from build123d import *

# Parameters (mm, degrees)
SKETCH2_W               = 9.652
SKETCH2_H               = 3.048
SKETCH2_W_2             = 3.048
SKETCH2_H_2             = 35.052
BOSS_EXTRUDE1_DEPTH     = 77.882279
SKETCH3_W               = 25.4
SKETCH3_H               = 76.2
SKETCH3_W_2             = 19.304
SKETCH3_H_2             = 70.104
BOSS_EXTRUDE2_DEPTH     = 50
CUT_EXTRUDE1_DEPTH      = 1
CUT_EXTRUDE1_DEPTH_BACK = 77.2
SKETCH5_W               = 25.4
SKETCH5_H               = 76.2
SKETCH5_W_2             = 19.304
SKETCH5_H_2             = 70.104
BOSS_EXTRUDE3_DEPTH     = 50
CUT_EXTRUDE2_DEPTH      = 1
CUT_EXTRUDE2_DEPTH_BACK = 77.2


with BuildPart() as part:
    # Sketch2 → Boss-Extrude1 (new body)
    with BuildSketch(Plane.XY):
        Polygon((-12.7, 0), (-9.652, 0), (-9.652, 35.052), (-9.652, 38.1), (-12.7, 38.1), align=None)
        with Locations((-4.826, 36.576)):
            Rectangle(SKETCH2_W, SKETCH2_H)
        Polygon((0, 38.1), (0, 35.052), (9.652, 35.052), (9.652, 0), (12.7, 0), (12.7, 38.1), align=None)
        with Locations((11.176, -17.526)):
            Rectangle(SKETCH2_W_2, SKETCH2_H_2)
        Polygon((-9.652, -35.052), (-9.652, 0), (-12.7, 0), (-12.7, -38.1), (0, -38.1), (0, -35.052), align=None)
        Polygon((9.652, -35.052), (0, -35.052), (0, -38.1), (12.7, -38.1), (12.7, -35.052), align=None)
    extrude(amount=BOSS_EXTRUDE1_DEPTH)

    # Sketch3 → Boss-Extrude2 (add)
    with BuildSketch(Plane(origin=(0, 0, 0), x_dir=(-1, 0, 0), z_dir=(0, 0, -1))):
        Rectangle(SKETCH3_W, SKETCH3_H)
        Rectangle(SKETCH3_W_2, SKETCH3_H_2, mode=Mode.SUBTRACT)
    extrude(amount=BOSS_EXTRUDE2_DEPTH)

    # Sketch4 → Cut-Extrude1 (cut, two sides)
    with BuildSketch(Plane(origin=(0, 38.1, 0), x_dir=(1, 0, 0), z_dir=(0, 1, 0))) as cut_extrude1_sk:
        Polygon((-119.729528752, 11.480724374), (-12.7, 1.217788135), (-12.7, 42.627933021), align=None)
        Polygon((-12.7, 1.217788135), (0, 0), (9.501519639, 49.088910403), (-12.7, 42.627933021), align=None)
        Polygon((12.7, -1.217788135), (119.729528752, -11.480724374), (127.176846342, 66.185439926), (-112.282211162, 89.146888673), (-119.729528752, 11.480724374), (-12.7, 42.627933021), (-12.7, 50), (12.7, 50), align=None)
        Polygon((0, 0), (12.7, -1.217788135), (12.7, 50), (-12.7, 50), (-12.7, 42.627933021), (9.501519639, 49.088910403), align=None)
    extrude(amount=CUT_EXTRUDE1_DEPTH, mode=Mode.SUBTRACT)
    extrude(cut_extrude1_sk.sketch, amount=-CUT_EXTRUDE1_DEPTH_BACK, mode=Mode.SUBTRACT)

    # Sketch5 → Boss-Extrude3 (add)
    with BuildSketch(Plane.XY.offset(77.882278635)):
        Rectangle(SKETCH5_W, SKETCH5_H)
        Rectangle(SKETCH5_W_2, SKETCH5_H_2, mode=Mode.SUBTRACT)
    extrude(amount=BOSS_EXTRUDE3_DEPTH)

    # Sketch6 → Cut-Extrude2 (cut, two sides)
    with BuildSketch(Plane.XZ.offset(38.1)) as cut_extrude2_sk:
        Polygon((-113.161207677, 166.450733215), (-103.71485858, 67.93718224), (-12.7, 124.967023668), (-12.7, 127.882278635), (12.7, 127.882278635), (12.7, 79.100066771), (103.71485858, 87.827375031), (94.268509483, 186.340926006), align=None)
        Polygon((-12.7, 124.967023668), (-103.71485858, 67.93718224), (-12.7, 76.6644905), align=None)
        Polygon((-12.7, 127.882278635), (-12.7, 124.967023668), (-9.501519639, 126.971189038), (0, 77.882278635), (12.7, 79.100066771), (12.7, 127.882278635), align=None)
        Polygon((-12.7, 124.967023668), (-12.7, 76.6644905), (0, 77.882278635), (-9.501519639, 126.971189038), align=None)
    extrude(amount=CUT_EXTRUDE2_DEPTH, mode=Mode.SUBTRACT)
    extrude(cut_extrude2_sk.sketch, amount=-CUT_EXTRUDE2_DEPTH_BACK, mode=Mode.SUBTRACT)


solid = part.part
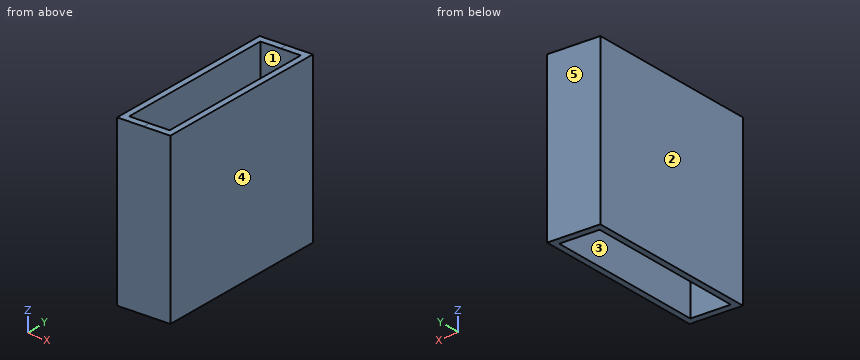
Input: part model. Units: mm. Frame: model coordinates. Face numbers are marked on the shaded views. A direction names the side the tool comes from. Give positions to 0.01 mm unless a question says otherwise; leave off trailing zeros. Order: outer loops, then holes, each group sorted by start corner. A loop starts at its lowest first (then second) coordinate and runs counter-clockwise, first axis right, second up. Notation, with made-up numbers: (22.25, 25) - (30.25, 25) arc R16 ccw to (30.25, 41) - close; hole circle Ø1 at (-4.75, 0). An arc over 180 degrees is marked (long way). Answer as a JSON object with one key per item and string values. Group by question number.
Q1. Cut plane B-B, the plane z = 68. Output: boundary loops of the cut face in (x, y).
Q2. Cut plane A-A, the plane y = 5.5. Output: boundary loops of the cut face in (x, z), then the cut area to 3 significant figures.
Q3. Cut plane C-C, the plane x = -1.75. Output: boundary loops of the cut face in (y, z).
Q4. Line query: probe 1 along X at (y, z) = (24, 75.5); probe 2 along Y at (x, z) = (1.5, 46.5); probe 3 along Z at (x, y) = (-4.5, 35.5). Output: solid intervals per line, ascending.
Q5. First-contact query: pin 1 Ø8 at (x, y) = (-6, -20) entering from -Z. Flat tip, straight axial feed; report the tip coordinate or a pass-through.
Q6. Mould query, pull axis X, two halves, no side actions, for the marked faces 3, 4 and 5. Classes: pulls with the +X half, pulls with the -X half, needs draft (parallel to the pull), parting line crosses it, or undercut.
Q7. Set-up query: the marked faces 1 and 2. Return all of +Z, -Z, +X, -X, +Y, -Y with unobstructed straight access to the full face (end or side cutting, diameter ignored); none if empty.
Results:
{
 "1": {"outline": "(-12.7, -38.1) - (12.7, -38.1) - (12.7, 38.1) - (-12.7, 38.1) - close; hole (-9.65, -35.05) - (9.65, -35.05) - (9.65, 35.05) - (-9.65, 35.05) - close"},
 "2": {"outline": "(-12.7, -1.22) - (-9.65, -0.93) - (-9.65, 76.96) - (-12.7, 76.66) - close; (9.65, 0.93) - (12.7, 1.22) - (12.7, 79.1) - (9.65, 78.81) - close", "area": "475 mm^2"},
 "3": {"outline": "(-38.1, -0.17) - (-35.05, -0.17) - (-35.05, 77.71) - (-38.1, 77.71) - close; (35.05, -0.17) - (38.1, -0.17) - (38.1, 77.71) - (35.05, 77.71) - close"},
 "4": {"probe 1": "-12.7 to -9.65, 9.65 to 12.7", "probe 2": "-38.1 to -35.05, 35.05 to 38.1", "probe 3": "-0.43 to 77.45"},
 "5": {"pin 1": "z = -0.96"},
 "6": {"face 3": "undercut", "face 4": "pulls with the +X half", "face 5": "needs draft"},
 "7": {"face 1": "+Z, -Z", "face 2": "+Z, -Z, -X, +Y, -Y"}
}
